For this review, take the finished solid that the model builds, in its own axes (mm). A direction names the side the tool comes from. Give positions to 0.01 mm unless a question says otherwise; leave off trailing zeros. Loops run counter-clockwise (first coordinate to the right, second up) from the corner with the lowest first, then second, coordinate; pieces in that order, holes last.
```python
from build123d import *

# Parameters (mm, degrees)
ESQUISSE1_R             = 15
ESQUISSE1_R_2           = 10
BOSS_EXTRU_1_DEPTH      = 180
BOSS_EXTRU_2_DEPTH      = 100
ESQUISSE3_W             = 17
ESQUISSE3_H             = 17
BOSS_EXTRU_3_DEPTH      = 20
ESQUISSE4_R             = 3.5
ENL_V_MAT_EXTRU_1_DEPTH = 20


with BuildPart() as part:
    # Esquisse1 → Boss.-Extru.1 (new body)
    with BuildSketch(Plane.XY):
        with Locations(Location((0, 0, 0), (0, 0, 180))):
            Circle(ESQUISSE1_R)
        with Locations(Location((0, 0, 0), (0, 0, 180))):
            Circle(ESQUISSE1_R_2, mode=Mode.SUBTRACT)
    extrude(amount=BOSS_EXTRU_1_DEPTH)

    # Esquisse2 → Boss.-Extru.2 (add)
    with BuildSketch(Plane(origin=(0, 0, 0), x_dir=(-1, 0, 0), z_dir=(0, 0, -1))):
        with BuildLine():
            Line((0, 15), (24, 15))
            ThreePointArc((24, 15), (39, 0), (24, -15))
            Line((24, -15), (0, -15))
            ThreePointArc((0, -15), (-15, 0), (0, 15))
        make_face()
    extrude(amount=-BOSS_EXTRU_2_DEPTH)

    # Esquisse3 → Boss.-Extru.3 (add)
    with BuildSketch(Plane(origin=(0, 0, 0), x_dir=(-1, 0, 0), z_dir=(0, 0, -1))):
        Rectangle(ESQUISSE3_W, ESQUISSE3_H)
    extrude(amount=BOSS_EXTRU_3_DEPTH)

    # Esquisse4 → Enlèv. mat.-Extru.1 (cut)
    with BuildSketch(Plane(origin=(0, 8.5, 0), x_dir=(1, 0, 0), z_dir=(0, 1, 0))):
        with Locations(Location((0, 10, 0), (0, 0, 180))):
            Circle(ESQUISSE4_R)
    extrude(amount=-ENL_V_MAT_EXTRU_1_DEPTH, mode=Mode.SUBTRACT)


solid = part.part
```
Item 1: Take a section at A-A on z = -10. Give the boundary of the cut face in (x, y).
Answer:
outline: (-8.5, -8.5) - (-3.5, -8.5) - (-3.5, 8.5) - (-8.5, 8.5) - close; (3.5, -8.5) - (8.5, -8.5) - (8.5, 8.5) - (3.5, 8.5) - close
Item 2: Take a section at D-D on x = -36. Give the boundary of the cut face in (y, z), and give its area (3 significant figures).
Answer:
outline: (-9, 0) - (9, 0) - (9, 100) - (-9, 100) - close
area: 1,800 mm2
Item 3: Take a section at C-C on z = 164. Give the boundary of the cut face in (x, y), and give its area (3 significant figures).
Answer:
outline: circle Ø30 at (0, 0); hole circle Ø20 at (0, 0)
area: 393 mm2
Item 4: Take a section at B-B on y = 0. Give the boundary of the cut face in (x, z).
Answer:
outline: (-39, 0) - (-8.5, 0) - (-8.5, -20) - (8.5, -20) - (8.5, 0) - (15, 0) - (15, 180) - (10, 180) - (10, 100) - (-10, 100) - (-10, 180) - (-15, 180) - (-15, 100) - (-39, 100) - close; hole circle Ø7 at (0, -10)
Item 5: Tool access review of faces 1 (the cylindrical face through (10, 0, 139)), 2 (the flat face through (-4, 8.5, -10)), 3 (the flat face through (-8.5, 0, -10)): name each direction out of +Z, -Z, +X, -X, +Y, -Y from which nothing blocks a thin tool from reaching the whole face with its end or side.
Answer:
face 1: +Z
face 2: -Z, +X, -X, +Y
face 3: -Z, -X, +Y, -Y
Item 6: The part is to be moulded in two halves that separate along Z. For faces 4 (the cylindrical face through (0.759, 0.119, -13.417)), 5 (the flat face through (-4, -8.5, -10)), 6 (the flat face through (0, 0, -20)), say which applies: released by +Z, released by -Z, zero draft, split by the parting line, or undercut.
Answer:
face 4: undercut
face 5: zero draft
face 6: released by -Z
Item 7: For L1, parallel to Z at x = 0, y = -4.5; L2, parallel to Z at x = -36, y = -3.5; L3, parallel to Z at x = 6.5, y = 0, list the stretches that pass through material, from the lowest coordinate up.
Answer:
L1: z = -20 to -13.5, -6.5 to 100
L2: z = 0 to 100
L3: z = -20 to 100
Item 8: Clearance check with flat-ended pins moving along their axes: pin 1 Ø3 at (y, z) = (-6.5, 78.5) entering from -X; pin 2 Ø2 at (y, z) = (5, 84) entering from -X; pin 3 Ø13.5 at (x, z) = (3.5, -12.5) entering from -Y; pin 4 Ø3 at (y, z) = (1.5, 84.5) entering from +X. State where each tip first meets the part, or that it passes through.
Answer:
pin 1: stops at x = -38.14
pin 2: stops at x = -38.46
pin 3: stops at y = -8.5
pin 4: stops at x = 15
